Could you check a few things on this model? Use its own coordinates, in mm. Round coordinates to 2 decimals unless told otherwise and drop trailing zeros. Write each loop counter-clockwise with the first axis right and the second up, starting at its lowest first coordinate (ties: lowest second). Pieces come first, ordered by that corner, then holes. Notation, with made-up numbers: (28, 83) -> (79, 83) arc R17 ccw to (79, 90) -> close; hole circle Ø9 at (40.25, 77.25). An arc over 180 degrees is marked (long way). Answer in a Markdown table with one row per item.
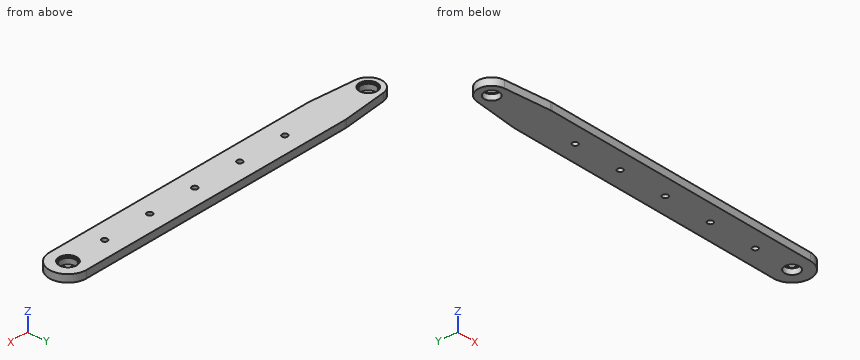
from build123d import *

# Parameters (mm, degrees)
EXTRUDE_1_DEPTH              = 4
HOLE_WIZARD_M5_1_D           = 8
HOLE_WIZARD_M5_1_CBORE_D     = 9.5
HOLE_WIZARD_M5_1_CBORE_DEPTH = 0.9
SKETCH_11_R                  = 1.5
CUT_EXTRUDE_1_DEPTH          = 1
CUT_EXTRUDE_1_DEPTH_BACK     = 5


with BuildPart() as part:
    # 草图1 → 凸台-拉伸1 (new body)
    with BuildSketch(Plane.XY):
        with BuildLine():
            Line((77.5, 10), (-77.5, 10))
            ThreePointArc((-77.5, 10), (-70.428932188, 7.071067812), (-67.5, 0))
            ThreePointArc((-67.5, 0), (-70.428932188, -7.071067812), (-77.5, -10))
            Line((-77.5, -10), (77.5, -10))
            ThreePointArc((77.5, -10), (87.5, 0), (77.5, 10))
        make_face()
        with BuildLine():
            ThreePointArc((-67.5, 0), (-70.428932188, 7.071067812), (-77.5, 10))
            ThreePointArc((-77.5, 10), (-78.000627751, 9.987460731), (-78.5, 9.949874371))
            ThreePointArc((-78.5, 9.949874371), (-87.5, 0), (-78.5, -9.949874371))
            ThreePointArc((-78.5, -9.949874371), (-78.000627751, -9.987460731), (-77.5, -10))
            ThreePointArc((-77.5, -10), (-70.428932188, -7.071067812), (-67.5, 0))
        make_face()
        with BuildLine():
            ThreePointArc((-78.5, -9.949874371), (-87.5, 0), (-78.5, 9.949874371))
            Line((-78.5, 9.949874371), (-103.25, 7.462405778))
            ThreePointArc((-103.25, 7.462405778), (-110, 0), (-103.25, -7.462405778))
            Line((-103.25, -7.462405778), (-78.5, -9.949874371))
        make_face()
    extrude(amount=EXTRUDE_1_DEPTH)

    # M5 六角头螺栓的柱形沉头孔1 (through all)
    with Locations(Plane.XY.offset(4)):
        with Locations((-102.5, 0), (77.5, 0)):
            CounterBoreHole(HOLE_WIZARD_M5_1_D / 2, HOLE_WIZARD_M5_1_CBORE_D / 2, HOLE_WIZARD_M5_1_CBORE_DEPTH)

    # 草图11 → 切除-拉伸1 (cut, two sides)
    with BuildSketch(Plane.XY.offset(4)) as cut_extrude_1_sk:
        with Locations((-52.5, 0)):
            Circle(SKETCH_11_R)
        with Locations((-25.5, 0)):
            Circle(SKETCH_11_R)
        with Locations((1.5, 0)):
            Circle(SKETCH_11_R)
        with Locations((28.5, 0)):
            Circle(SKETCH_11_R)
        with Locations((55.5, 0)):
            Circle(SKETCH_11_R)
    extrude(amount=CUT_EXTRUDE_1_DEPTH, mode=Mode.SUBTRACT)
    extrude(cut_extrude_1_sk.sketch, amount=-CUT_EXTRUDE_1_DEPTH_BACK, mode=Mode.SUBTRACT)


solid = part.part
1) For pin 1 (2.5 mm diameter, centred on x = -25.5, y = 0, fed in from -Z); pin 2 (1 mm diameter, centred on y = -2.5, z = 2.5, fed in from -X), each with a flat end and sliding along its axis, tell me the tip position at first contact or that it passes through.
Findings:
| item | result |
|---|---|
| pin 1 | passes through |
| pin 2 | stops at x = -109.73 |
2) Please list where these lines run through material, in increasing order: line 1 (Y direction, x = -52.5, z = 1.5); line 2 (X direction, y = -2.75, z = 3.5); line 3 (Y direction, x = 77.5, z = 2.45).
Findings:
| item | result |
|---|---|
| line 1 | y = -10 to -1.5, 1.5 to 10 |
| line 2 | x = -109.48 to -106.37, -98.63 to 73.63, 81.37 to 87.11 |
| line 3 | y = -10 to -4, 4 to 10 |
3) Imagine slicing it at A-A, the plane z = 1.25. Please give me the cut outline in (x, y).
Findings:
| item | result |
|---|---|
| outline | (-103.25, -7.46) -> (-78.5, -9.95) arc R10 ccw to (-77.5, -10) -> (77.5, -10) arc R10 ccw to (77.5, 10) -> (-77.5, 10) arc R10 ccw to (-78.5, 9.95) -> (-103.25, 7.46) arc R7.5 ccw to start; hole circle Ø8 at (-102.5, 0); hole circle Ø3 at (-52.5, 0); hole circle Ø3 at (-25.5, 0); hole circle Ø3 at (1.5, 0); hole circle Ø3 at (28.5, 0); hole circle Ø3 at (55.5, 0); hole circle Ø8 at (77.5, 0) |
